The model under review builds one solid part; all positions refer to its coordinate system, in mm. A direction names the side the tool comes from. Round coordinates to 2 decimals unless told otherwise and drop trailing zeros. Write each loop counter-clockwise with the first axis right and the second up, starting at its lowest first coordinate (ties: lowest second). Pieces come first, ordered by that corner, then holes. Notation, with made-up numbers: (-24, 10.25) -> (30, 10.25) arc R22 ccw to (30, 28.25) -> close; hole circle Ø2 at (-29, 49.25). An arc over 180 degrees is marked (long way). Answer as a JSON object with one key per item and string values. Group by question number.
1) We need section B-B, the plane x = 14.5. Write out the cut boundary in (y, z), then the cut area to 3 significant figures.
2) Machinability: for faces 1 (the flat face through (66, 2, -46)), 2 (the cylindrical face through (14.981, 1.578, -47.674)), which of the approach directions +Z, -Z, +X, -X, +Y, -Y give a long, thin tool a straight path to every point of the face, cutting with its end or side? Answer none if there is none.
3) We need section C-C, the plane y = 0.7. Write out the cut boundary in (x, z).
4) To check wall thickness, follow probe 1 along X at (y, z) = (2.55, -7); probe 2 along Z at (x, y) = (13.5, 0.5); probe 3 along X at (y, z) = (1.1, -49.2). State the ranges of each line that lie inside material, in increasing order. Write a range as [from, to].
5) We need section D-D, the plane z = -49.2. Write out the cut boundary in (x, y).
6) Mouldability with a two-part tool opening along X and no side actions: class faces 3 (the cylindrical face through (67.586, 1.578, -35.308)), 4 (the flat face through (0, 2, -26)), 5 (the flat face through (34, 3.2, -26)) as pulls with the +X half, pulls with the -X half, needs draft (parallel to the pull), parting line crosses it, or undercut.
7) Insertion check: pin 1 Ø4 at (x, z) = (66, -35.1) entering from +Y; pin 2 Ø2.5 at (x, z) = (14.5, -49.2) entering from -Y; pin 3 Ø1.6 at (y, z) = (2.5, -46) entering from +X. Each pin has a flat end and moves straight along its axis. Give the tip position at first contact, or say it passes through.
8) We need section A-A, the plane z = -7. Write out the cut boundary in (x, y), then the cut area to 3 significant figures.
from build123d import *

# Parameters (mm, degrees)
CROQUIS1_R              = 1.6
SALIENTE_EXTRUIR1_DEPTH = 3.2


with BuildPart() as part:
    # Croquis1 → Saliente-Extruir1 (new body)
    with BuildSketch(Plane(origin=(0, 0, 0), x_dir=(1, 0, 0), z_dir=(0, 1, 0))):
        Polygon((0, 0), (66, 0), (69.2, 3.2), (69.2, 37.2), (66, 40.4), (66, 51.5), (0, 51.5), align=None)
        with Locations(Location((14.5, 49.2, 0), (0, 0, 270))):
            Circle(CROQUIS1_R, mode=Mode.SUBTRACT)
        with Locations(Location((14.5, 1.9, 0), (0, 0, 270))):
            Circle(CROQUIS1_R, mode=Mode.SUBTRACT)
        with Locations(Location((66, 35.1, 0), (0, 0, 270))):
            Circle(CROQUIS1_R, mode=Mode.SUBTRACT)
        with Locations(Location((66, 7, 0), (0, 0, 270))):
            Circle(CROQUIS1_R, mode=Mode.SUBTRACT)
    extrude(amount=SALIENTE_EXTRUIR1_DEPTH)


solid = part.part
Here are the results:
{
 "1": {"outline": "(0, -51.5) -> (3.2, -51.5) -> (3.2, -50.8) -> (0, -50.8) -> close; (0, -47.6) -> (3.2, -47.6) -> (3.2, -3.5) -> (0, -3.5) -> close; (0, -0.3) -> (3.2, -0.3) -> (3.2, 0) -> (0, 0) -> close", "area": "144 mm^2"},
 "2": {"face 1": "-Z, +X, +Y, -Y", "face 2": "+Y, -Y"},
 "3": {"outline": "(0, -51.5) -> (66, -51.5) -> (66, -40.4) -> (69.2, -37.2) -> (69.2, -3.2) -> (66, 0) -> (0, 0) -> close; hole circle Ø3.2 at (14.5, -49.2); hole circle Ø3.2 at (14.5, -1.9); hole circle Ø3.2 at (66, -35.1); hole circle Ø3.2 at (66, -7)"},
 "4": {"probe 1": "x = [0, 64.4], [67.6, 69.2]", "probe 2": "z = [-51.5, -50.45], [-47.95, -3.15], [-0.65, 0]", "probe 3": "x = [0, 12.9], [16.1, 66]"},
 "5": {"outline": "(0, 0) -> (12.9, 0) -> (12.9, 3.2) -> (0, 3.2) -> close; (16.1, 0) -> (66, 0) -> (66, 3.2) -> (16.1, 3.2) -> close"},
 "6": {"face 3": "undercut", "face 4": "pulls with the -X half", "face 5": "needs draft"},
 "7": {"pin 1": "stops at y = 3.2", "pin 2": "passes through", "pin 3": "stops at x = 66"},
 "8": {"outline": "(0, 0) -> (64.4, 0) -> (64.4, 3.2) -> (0, 3.2) -> close; (67.6, 0) -> (69.2, 0) -> (69.2, 3.2) -> (67.6, 3.2) -> close", "area": "211 mm^2"}
}
